```python
from build123d import *

# Parameters (mm, degrees)
SKETCH1_R           = 13.25
SKETCH1_R_2         = 6
BOSS_EXTRUDE1_DEPTH = 5
SKETCH2_R           = 1.25
CUT_EXTRUDE1_DEPTH  = 6


with BuildPart() as part:
    # Sketch1 → Boss-Extrude1 (new body)
    with BuildSketch(Plane.XY):
        Circle(SKETCH1_R)
        Circle(SKETCH1_R_2, mode=Mode.SUBTRACT)
        with BuildLine():
            Line((100, 13.25), (0, 13.25))
            ThreePointArc((0, 13.25), (9.369164851, 9.369164851), (13.25, 0))
            ThreePointArc((13.25, 0), (9.369164851, -9.369164851), (0, -13.25))
            Line((0, -13.25), (100, -13.25))
            ThreePointArc((100, -13.25), (86.75, 0), (100, 13.25))
        make_face()
        with BuildLine():
            Line((80, -3), (50, -3))
            Line((50, -3), (20, -3))
            ThreePointArc((20, -3), (17, 0), (20, 3))
            Line((20, 3), (50, 3))
            Line((50, 3), (80, 3))
            ThreePointArc((80, 3), (82.121320344, 2.121320344), (83, 0))
            ThreePointArc((83, 0), (82.121320344, -2.121320344), (80, -3))
        make_face(mode=Mode.SUBTRACT)
        with Locations((100, 0)):
            Circle(SKETCH1_R)
        with Locations((100, 0)):
            Circle(SKETCH1_R_2, mode=Mode.SUBTRACT)
    extrude(amount=BOSS_EXTRUDE1_DEPTH)

    # Sketch2 → Cut-Extrude1 (cut, through all)
    with BuildSketch(Plane.XY.offset(5)):
        with Locations((100, 10.25)):
            Circle(SKETCH2_R)
        with Locations((108.876760389, 5.125)):
            Circle(SKETCH2_R)
        with Locations((8.876760389, 5.125)):
            Circle(SKETCH2_R)
        with Locations((8.876760389, -5.125)):
            Circle(SKETCH2_R)
        with Locations((-8.876760389, 5.125)):
            Circle(SKETCH2_R)
        with Locations((-8.876760389, -5.125)):
            Circle(SKETCH2_R)
        with Locations((0, -10.25)):
            Circle(SKETCH2_R)
        with Locations((0, 10.25)):
            Circle(SKETCH2_R)
        with Locations((91.123239611, 5.125)):
            Circle(SKETCH2_R)
        with Locations((108.876760389, -5.125)):
            Circle(SKETCH2_R)
        with Locations((100, -10.25)):
            Circle(SKETCH2_R)
        with Locations((91.123239611, -5.125)):
            Circle(SKETCH2_R)
    extrude(amount=-CUT_EXTRUDE1_DEPTH, mode=Mode.SUBTRACT)


solid = part.part
```
Here's how the part is built. I have some questions about the finished solid (model axes, mm). A direction names the side the tool comes from. Coordinates: 2 decimals unless noted, no trailing zeros. Loops run counter-clockwise (first coordinate to the right, second up) from the corner with the lowest first, then second, coordinate; pieces in that order, holes last. Notation, with made-up numbers: M -9,-1 L 7,-1 A14 cw 7,17 Z; hole C 45.25,35.5 d5. An arc over 180 degrees is marked long. One line per item, written item: value.
1. On a 3-axis mill with a long thin cutter (end or side, diameter ignored), from which of +Z, -Z, +X, -X, +Y, -Y can I reach the whole of each face in a straight line? I mean faces 1 (the flat face through (50, -3, 2)), 2 (the flat face through (49, 6, 0)). Say none if no direction works.
Geometry says:
face 1: +Z, -Z
face 2: -Z, +X, -X, +Y, -Y
2. Will this pin go through, and if not, where does the flat tip stop? pin 1 Ø2 at (x, y) = (99, -3) entering from -Z.
Geometry says:
pin 1: passes through
3. Thinking about a two-plate mould opening in X: for faces 3 (the cylindrical face through (113.247, -0.291, 2.465)), 4 (the flat face through (49, 6, 5)), 5 (the cylindrical face through (-13.247, 0.291, 2.465)), 6 (the cylindrical face through (101.2, -9.9, 2.5)), which applies, +X half, -X half, draft (parallel to the pull), parting line (faces both ways), or undercut?
Geometry says:
face 3: +X half
face 4: draft
face 5: -X half
face 6: undercut
4. Imagine slicing it at C-C (z = 2.1). State how many separate pieces and enclosed holes the cut face has, and give its area (3 significant figures).
Geometry says:
separate pieces: 1
enclosed holes: 15
area: 2,530 mm2
5. Imagine slicing it at D-D (y = -10.25). List the corners of the cut face in (x, z) for me.
Geometry says:
outline: M -8.4,0 L -1.25,0 L -1.25,5 L -8.4,5 Z; M 1.25,0 L 98.75,0 L 98.75,5 L 1.25,5 Z; M 101.25,0 L 108.4,0 L 108.4,5 L 101.25,5 Z
6. Imagine slicing it at B-B (y = -1.5). List the corners of the cut face in (x, z) for me.
Geometry says:
outline: M -13.16,0 L -5.81,0 L -5.81,5 L -13.16,5 Z; M 5.81,0 L 17.4,0 L 17.4,5 L 5.81,5 Z; M 82.6,0 L 94.19,0 L 94.19,5 L 82.6,5 Z; M 105.81,0 L 113.16,0 L 113.16,5 L 105.81,5 Z
7. Imagine slicing it at A-A (x = 44.5). List the corners of the cut face in (y, z) for me, and give its area (4 significant figures).
Geometry says:
outline: M -13.25,0 L -3,0 L -3,5 L -13.25,5 Z; M 3,0 L 13.25,0 L 13.25,5 L 3,5 Z
area: 102.5 mm2
8. Please list where these lines run through material, in increasing order: probe 1 along Y at (x, z) = (9, 1.05); probe 2 along Y at (x, z) = (71.5, 0.4).
Geometry says:
probe 1: y = -13.25 to -6.37, -3.88 to 3.88, 6.37 to 13.25
probe 2: y = -13.25 to -3, 3 to 13.25
